Can you work these out from the model? Positions are in its coordinate system, mm. A direction names the side the tool comes from. Give positions to 0.01 mm unless a question says otherwise; leave off trailing zeros. Order: outer loops, then holes, each group sorted by start corner. A loop starts at its lowest first (then second) coordinate and runs counter-clockwise, first axis right, second up.
Item 1: I want a section at D-D, the plane x = 10.5. Write out the boundary of the cut face in (y, z).
Item 2: Which directions (+Z, -Z, +X, -X, +Y, -Y) give clear straight access to the entire face, cutting with the end or side of a thin tool? Please do faces 1 (the flat face through (2, -2, 9.9)), 2 (the cylindrical face through (0.21, 7.07, 2.95)).
Item 3: I want a section at B-B, the plane x = -17.01. Write out the boundary of the cut face in (y, z), then the cut area to 3 significant figures.
Item 4: I want a section at C-C, the plane z = 12. Write out the boundary of the cut face in (x, y), then the cut area to 3 significant figures.
Item 5: I'm going to push flat-ended pins straight in: pin 1 Ø4 at (x, y) = (1, 0) entering from -Z; pin 2 Ø2.5 at (x, z) = (10, 14.5) entering from +Y; pin 3 Ø1.5 at (x, y) = (5, -2) entering from +Z. Where does each tip first touch, or does it pass through?
Item 6: I want a section at A-A, the plane y = -0.76. Count the separate pieces of the cut face and the enclosed holes in it, then the cut area to 3 significant figures.
Item 7: If we mould it in two halves opening along X, with no side actions, what happens to faces 3 (the flat face through (31, 3, 22)), 4 (the cylindrical face through (12.33, 3.4, 4.29)), 5 (the flat face through (8, -3.75, 11))? For each: +X half, -X half, draft (parallel to the pull), parting line (faces both ways), or undercut.
Item 8: If I drill on line 1 along Y through (x, z) = (-17.01, 6.75); line 2 along X through (y, z) = (0, 3.2); line 3 along Z through (x, y) = (21.75, 7.5), over which ranges is the centre line in solid material (lowest first)?
```python
from build123d import *

# Parameters (mm, degrees)
F0_W         = 47
F0_H         = 14.5
F0_R         = 1.3
F0_R_2       = 2
F1_DEPTH     = 19
F4_DEPTH     = 9.9
F5_R         = 1.5
F5_R_2       = 1.4
F6_DEPTH     = 14.5
F7_DEPTH     = 10
F8_W         = 6
F8_H         = 14.5
F9_DEPTH     = 10
F10_R        = 2
F11_DEPTH    = 6
F12_T1_DEPTH = 29.5
F14_DEPTH    = 2


# Not quite as in the source:
# - a fillet or chamfer that OpenCascade refuses, or shapes differently, is made with other operations: its cross-section is extruded or revolved along the edge and cut away or added


with BuildPart() as f1:
    # F0 (on Top) → F1 (new body)
    with BuildSketch(Plane.XY):
        with Locations((3.5, 3.5)):
            Rectangle(F0_W, F0_H)
        with Locations((-17.01, -0.76)):
            Circle(F0_R, mode=Mode.SUBTRACT)
        Circle(F0_R_2, mode=Mode.SUBTRACT)
        with Locations((-17.01, 7.76)):
            Circle(F0_R, mode=Mode.SUBTRACT)
    extrude(amount=F1_DEPTH)

    # F2 (on face) → F3 (revolve, cut)
    with BuildSketch(Plane.XZ.offset(3.75)):
        Polygon((0, 9.93), (-7.995, 9.93), (-7.995, 5.98), (-5.995, 5.98), (-5.995, 0), (0, 0), align=None)
    revolve(axis=Axis((0, 0, 0), (0, 0, 1)), mode=Mode.SUBTRACT)

    # F4 (cut): a face of the model
    f4_faces = [f1.faces().sort_by_distance(p)[0] for p in [
        (0, 3.6439339828, 0),
    ]]
    extrude(f4_faces, amount=-F4_DEPTH, mode=Mode.SUBTRACT)

    # F5 (on face) → F6 (cut, through all)
    with BuildSketch(Plane.XZ.offset(3.75)):
        with Locations((-9.25, 12)):
            Circle(F5_R)
        with Locations((-10.5055273842, 3.7)):
            Circle(F5_R_2)
        with Locations((10.9938158954, 3.8680432901)):
            Circle(F5_R_2)
        with Locations((21.75, 12)):
            Circle(F5_R)
    extrude(amount=-F6_DEPTH, mode=Mode.SUBTRACT)

    # F7 (add): a face of the model
    f7_faces = [f1.faces().sort_by_distance(p)[0] for p in [
        (27, 3.5, 9.5),
    ]]
    extrude(f7_faces, amount=F7_DEPTH)

    # F8 (on face) → F9 (join)
    with BuildSketch(Plane.XY.offset(19)):
        with Locations((34, 3.5)):
            Rectangle(F8_W, F8_H)
    extrude(amount=F9_DEPTH)

    # F10 (on face) → F11 (cut, through all)
    with BuildSketch(Plane.YZ.offset(37)):
        with Locations((0, 24.5)):
            Circle(F10_R)
    extrude(amount=-F11_DEPTH, mode=Mode.SUBTRACT)

    # F12: fillet of radius 3 on 2 edges, made by hand

    # F12_s2 → F12_t1 (cut)
    with BuildSketch(Plane.XZ.offset(-18.25)):
        with BuildLine():
            ThreePointArc((31, 26), (31.8786796564, 28.1213203436), (34, 29))
            Line((34, 29), (31, 29))
            Line((31, 29), (31, 26))
        make_face()
        with BuildLine():
            ThreePointArc((34, 29), (36.1213203436, 28.1213203436), (37, 26))
            Line((37, 26), (37, 29))
            Line((37, 29), (34, 29))
        make_face()
    extrude(amount=F12_T1_DEPTH, mode=Mode.SUBTRACT)

    # F13 (on face) → F14 (cut)
    with BuildSketch(Plane(origin=(0, 10.75, 0), x_dir=(-1, 0, 0), z_dir=(0, 1, 0))):
        with BuildLine():
            Line((7.2936857888, 19), (-18.2936857888, 19))
            ThreePointArc((-18.2936857888, 19), (-5.5, 11.3063278591), (7.2936857888, 19))
        make_face()
    extrude(amount=-F14_DEPTH, mode=Mode.SUBTRACT)


solid = f1.part
```
Results list:
1. outline: (-3.75, 0) - (10.75, 0) - (10.75, 2.56) - (-3.75, 2.56) - close; (-3.75, 5.18) - (10.75, 5.18) - (10.75, 12.2) - (8.75, 12.2) - (8.75, 19) - (-3.75, 19) - close
2. face 1: -Z, -Y
2. face 2: -Z
3. outline: (-3.75, 0) - (-2.06, 0) - (-2.06, 19) - (-3.75, 19) - close; (0.54, 0) - (6.46, 0) - (6.46, 19) - (0.54, 19) - close; (9.06, 0) - (10.75, 0) - (10.75, 19) - (9.06, 19) - close
3. area: 177 mm2
4. outline: (-20, -3.75) - (-10.75, -3.75) - (-10.75, 10.75) - (-20, 10.75) - close; (-7.75, -3.75) - (20.25, -3.75) - (20.25, 10.75) - (9.93, 10.75) - (9.93, 8.75) - (1.07, 8.75) - (1.07, 10.75) - (-7.75, 10.75) - close; (23.25, -3.75) - (37, -3.75) - (37, 10.75) - (23.25, 10.75) - close; hole circle Ø2.6 at (-17.01, -0.76); hole circle Ø2.6 at (-17.01, 7.76); hole circle Ø4 at (0, 0)
4. area: 699 mm2
5. pin 1: stops at z = 9.9
5. pin 2: stops at y = 8.75
5. pin 3: stops at z = 19
6. separate pieces: 4
6. enclosed holes: 4
6. area: 854 mm2
7. face 3: -X half
7. face 4: undercut
7. face 5: draft
8. line 1: y = -3.75 to -2.06, 0.54 to 6.46, 9.06 to 10.75
8. line 2: x = -20 to -18.06, -15.96 to -11.81, -9.2 to -7.07, 7.07 to 9.76, 12.22 to 37
8. line 3: z = 0 to 10.5, 13.5 to 19
